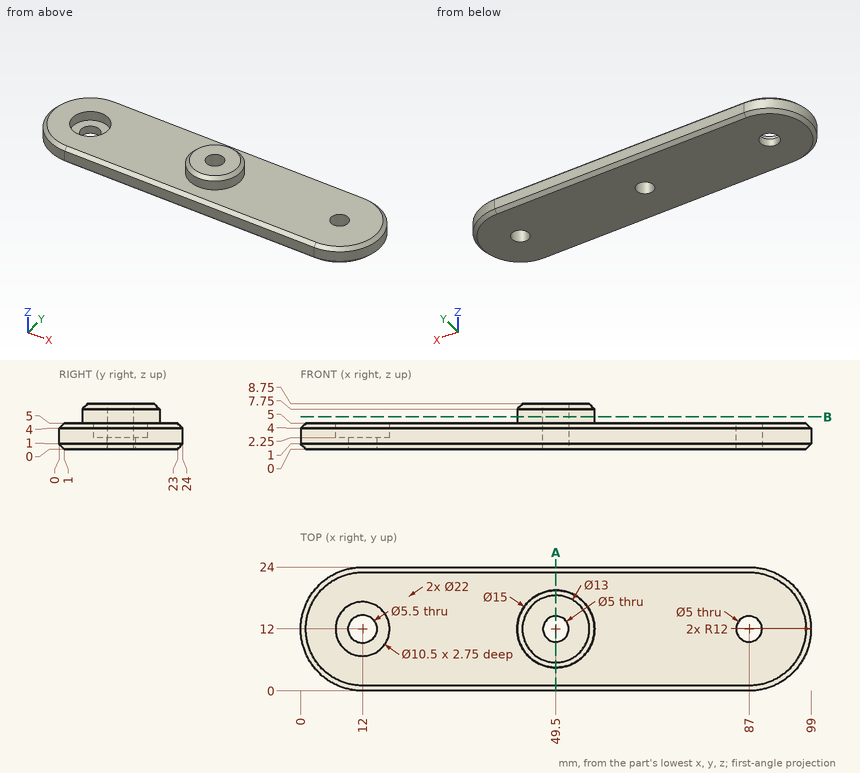
Print and shaded views of the part. All mm, measured from the part's lowest x, y and z. Round coordinates to 2 decimals unless told otherwise and drop trailing zeros. Write each loop counter-clockwise with the first axis right and the second up, starting at its lowest first coordinate (ties: lowest second). Pieces come first, ordered by that corner, then holes. Notation, with made-up numbers: M 1.25,74.25 L 15.25,74.25 A10 cw 15.25,84.25 Z; hole C 26.25,73.5 d2. An arc over 180 degrees is marked long. Use a Markdown table: item, result. Add a question column.
1. Flat gauge pins, fed straight in: P1, Ø4.5, axis at x = 12, y = 12, coming from the -Z side; P2, Ø1, axis at x = 66.5, y = 5.5, coming from the +Z side; P3, Ø9.5, axis at x = 12, y = 12, coming from the +Z side; P4, Ø1, axis at y = 3, z = 2, coming from the +X side. Where does each tip first touch, or does it go through?
2. Slice it at A-A on x = 49.5. Give the cut face in (y, z), then the cut area to 4 significant figures.
3. Drill centre lines: probe 1 along Y at (x, z) = (12, 3.3); probe 2 along Y at (x, z) = (12, 1.4); probe 3 along Z at (x, y) = (59.5, 3.25). Where is each one in solid material? Low to high.
4. Slice it at B-B on z = 6.25. Give the cut face in (x, y).
Reply:
| question | item | result |
|---|---|---|
| 1 | P1 | passes through |
| 1 | P2 | stops at z = 5 |
| 1 | P3 | stops at z = 2.25 |
| 1 | P4 | stops at x = 95.47 |
| 2 | outline | M 0,1 L 1,0 L 9.5,0 L 9.5,8.75 L 5.5,8.75 L 4.5,7.75 L 4.5,5 L 1,5 L 0,4 Z; M 14.5,0 L 23,0 L 24,1 L 24,4 L 23,5 L 19.5,5 L 19.5,7.75 L 18.5,8.75 L 14.5,8.75 Z |
| 2 | area | 129.5 mm^2 |
| 3 | probe 1 | y = 0 to 6.75, 17.25 to 24 |
| 3 | probe 2 | y = 0 to 9.25, 14.75 to 24 |
| 3 | probe 3 | z = 0 to 5 |
| 4 | outline | C 49.5,12 d15; hole C 49.5,12 d5 |
